Read the model definition and answer for the solid it produces. Units are mm, in the model's axes. Face numbers are marked on the shaded views. Give positions to 0.01 mm unless a question says otherwise; leave off trailing zeros. Order: outer loops, then holes, each group sorted by start corner. A loop starts at its lowest first (then second) coordinate and runs counter-clockwise, first axis right, second up. Notation, with made-up numbers: M -38.5,63.25 L -16.5,63.25 A20 cw -16.5,94.25 Z; hole C 29,65.25 d6. An arc over 180 degrees is marked long. One line per item, written item: value.
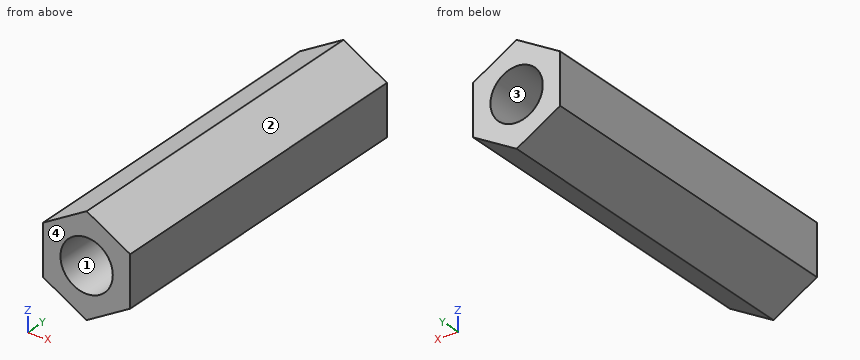
from build123d import *

# Parameters (mm, degrees)
BOSS_EXTRUDE1_DEPTH = 40
SKETCH3_R           = 3
CUT_EXTRUDE1_DEPTH  = 12
SKETCH4_R           = 3
CUT_EXTRUDE2_DEPTH  = 12


with BuildPart() as part:
    # Sketch1 → Boss-Extrude1 (new body)
    with BuildSketch(Plane(origin=(0, 0, 0), x_dir=(1, 0, 0), z_dir=(0, 1, 0))):
        Polygon((0, -5.773502692), (5, -2.886751346), (5, 2.886751346), (0, 5.773502692), (-5, 2.886751346), (-5, -2.886751346), align=None)
    extrude(amount=BOSS_EXTRUDE1_DEPTH)

    # Sketch3 → Cut-Extrude1 (cut)
    with BuildSketch(Plane.XZ):
        Circle(SKETCH3_R)
    extrude(amount=-CUT_EXTRUDE1_DEPTH, mode=Mode.SUBTRACT)

    # Sketch4 → Cut-Extrude2 (cut)
    with BuildSketch(Plane(origin=(0, 40, 0), x_dir=(1, 0, 0), z_dir=(0, 1, 0))):
        Circle(SKETCH4_R)
    extrude(amount=-CUT_EXTRUDE2_DEPTH, mode=Mode.SUBTRACT)


solid = part.part
1) Find section D-D, the plane x = -0.75. Write down the section's boundary in (y, z), plus the area to 3 significant figures.
Reported:
outline: M 0,-5.34 L 40,-5.34 L 40,-2.9 L 28,-2.9 L 28,2.9 L 40,2.9 L 40,5.34 L 0,5.34 L 0,2.9 L 12,2.9 L 12,-2.9 L 0,-2.9 Z
area: 288 mm^2
2) Consider probe 1 along Z at (x, y) = (0, 5); probe 2 along X at (y, z) = (37.25, 0); probe 3 along Y at (x, z) = (0.25, -2.25). Determine where each line is inside the solid, lowest interval first.
Reported:
probe 1: z = -5.77 to -3, 3 to 5.77
probe 2: x = -5 to -3, 3 to 5
probe 3: y = 12 to 28
3) Find section C-C, the plane y = 17.5. Write down the section's boundary in (x, z).
Reported:
outline: M -5,-2.89 L 0,-5.77 L 5,-2.89 L 5,2.89 L 0,5.77 L -5,2.89 Z
4) Each of these flat-tipped pins is pushed along its axis until it touches: pin 1 Ø5 at (x, y) = (-1, 23.5) entering from -Z; pin 2 Ø3.5 at (x, z) = (0, 0) entering from -Y; pin 3 Ø6 at (x, z) = (1.5, 0) entering from +Y. Where does it stop, or does it pass through?
Reported:
pin 1: stops at z = -5.77
pin 2: stops at y = 12
pin 3: stops at y = 40
5) Find section A-A, the plane y = 5. Write down the section's boundary in (x, z), plus the area to 3 significant figures.
Reported:
outline: M -5,-2.89 L 0,-5.77 L 5,-2.89 L 5,2.89 L 0,5.77 L -5,2.89 Z; hole C 0,0 d6
area: 58.3 mm^2
6) Determine the mould class of the marked faces 1, 2, 3 and 4 for opening direction Z: +Z half, -Z half, draft (parallel to the pull), parting line (faces both ways), or undercut.
Reported:
face 1: undercut
face 2: +Z half
face 3: undercut
face 4: draft
7) Find section B-B, the plane z = 0. Write down the section's boundary in (x, y).
Reported:
outline: M -5,0 L -3,0 L -3,12 L 3,12 L 3,0 L 5,0 L 5,40 L 3,40 L 3,28 L -3,28 L -3,40 L -5,40 Z
